from build123d import *

# Parameters (mm, degrees)
F1_DEPTH = 193.04
F2_W     = 122.8137016296
F2_H     = 78.0344456434
F3_DEPTH = 25.4


# Not quite as in the source:
# - a feature names something its author has since deleted; it is built from what else it names


with BuildPart() as f1:
    # F0 (on Right) → F1 (new body)
    with BuildSketch(Plane.YZ):
        Polygon((-52.5168515742, 56.4679652452), (-52.5168515742, -44.9438914657), (58.7727762759, -44.9438914657), (58.7727762759, 56.4679652452), (0, 90.0208726525), align=None)
    extrude(amount=F1_DEPTH)

    # F2 (on Top) → F3 (join)
    with BuildSketch(Plane.XY):
        with Locations((-2.963334322, -2.6340745389)):
            Rectangle(F2_W, F2_H)
    extrude(amount=F3_DEPTH)


solid = f1.part
The model under review builds one solid part; all positions refer to its coordinate system, in mm. A direction names the side the tool comes from. Round coordinates to 2 decimals unless told otherwise and drop trailing zeros. Order: outer loops, then holes, each group sorted by start corner. A loop starts at its lowest first (then second) coordinate and runs counter-clockwise, first axis right, second up. Notation, with made-up numbers: (-3, 48) -> (9, 48) arc R16 cw to (9, 58) -> close; hole circle Ø2 at (65, -39). An arc over 180 degrees is marked (long way). Return JSON: item names as keys, results as strings.
1. Take a section at A-A (x = 162.5). Write out the cut boundary in (y, z), then the cut area to 3 significant figures.
Answer block:
{"outline": "(-52.52, -44.94) -> (58.77, -44.94) -> (58.77, 56.47) -> (0, 90.02) -> (-52.52, 56.47) -> close", "area": "13,200 mm²"}
2. Insertion check: P1, Ø20.5, axis at x = -30, z = 9, coming from the -Y side; P2, Ø7.5, axis at x = -38.5, z = 8, coming from the +Y side; P3, Ø1.5, axis at y = -24, z = -29, coming from the -X side. Each pin has a flat end and moves straight along its axis. Give the tip position at first contact, or say it passes through.
Answer block:
{"P1": "stops at y = -41.65", "P2": "stops at y = 36.38", "P3": "stops at x = 0"}
3. For L1, parallel to X at y = 48.5, z = 60; L2, parallel to Y at x = -8.5, z = 13; L3, parallel to Z at x = -8, y = 0, list the stretches that pass through material, from the lowest coordinate up. Write a range as [from, to].
Answer block:
{"L1": "x = [0, 193.04]", "L2": "y = [-41.65, 36.38]", "L3": "z = [0, 25.4]"}
4. Take a section at C-C (y = 28). Write out the cut boundary in (x, z).
Answer block:
{"outline": "(-64.37, 0) -> (0, 0) -> (0, -44.94) -> (193.04, -44.94) -> (193.04, 74.04) -> (0, 74.04) -> (0, 25.4) -> (-64.37, 25.4) -> close"}
5. The part is to be moulded in two halves that separate along Y. For faces 1 (the face through (95, -52.517, 6)), 2 (the face through (-33, 36.383, 13)), 3 (the face through (-64.37, -3, 13)), say which applies: +Y half, -Y half, draft (parallel to the pull), parting line (faces both ways), or undercut.
Answer block:
{"face 1": "-Y half", "face 2": "+Y half", "face 3": "draft"}
6. For faces 4 (the face through (-33, -2, 25.4)), 5 (the face through (95, 2, -44.944)), 6 (the face through (-33, -41.651, 13)), 7 (the face through (-33, -2, 0)), list the 3-axis set-ups (+Z, -Z, +X, -X, +Y, -Y) from which the entire face can be reached by the end or side of a thin tool; tool diameter is ignored.
Answer block:
{"face 4": "+Z, -X, +Y, -Y", "face 5": "-Z, +X, -X, +Y, -Y", "face 6": "+Z, -Z, -X, -Y", "face 7": "-Z, -X, +Y, -Y"}
7. Take a section at B-B (z = 10). Write out the cut boundary in (x, y), then the cut area to 3 significant figures.
Answer block:
{"outline": "(-64.37, -41.65) -> (0, -41.65) -> (0, -52.52) -> (193.04, -52.52) -> (193.04, 58.77) -> (0, 58.77) -> (0, 36.38) -> (-64.37, 36.38) -> close", "area": "26,500 mm²"}
8. Take a section at D-D (z = 44.5). Write out the cut boundary in (x, y).
Answer block:
{"outline": "(0, -52.52) -> (193.04, -52.52) -> (193.04, 58.77) -> (0, 58.77) -> close"}
